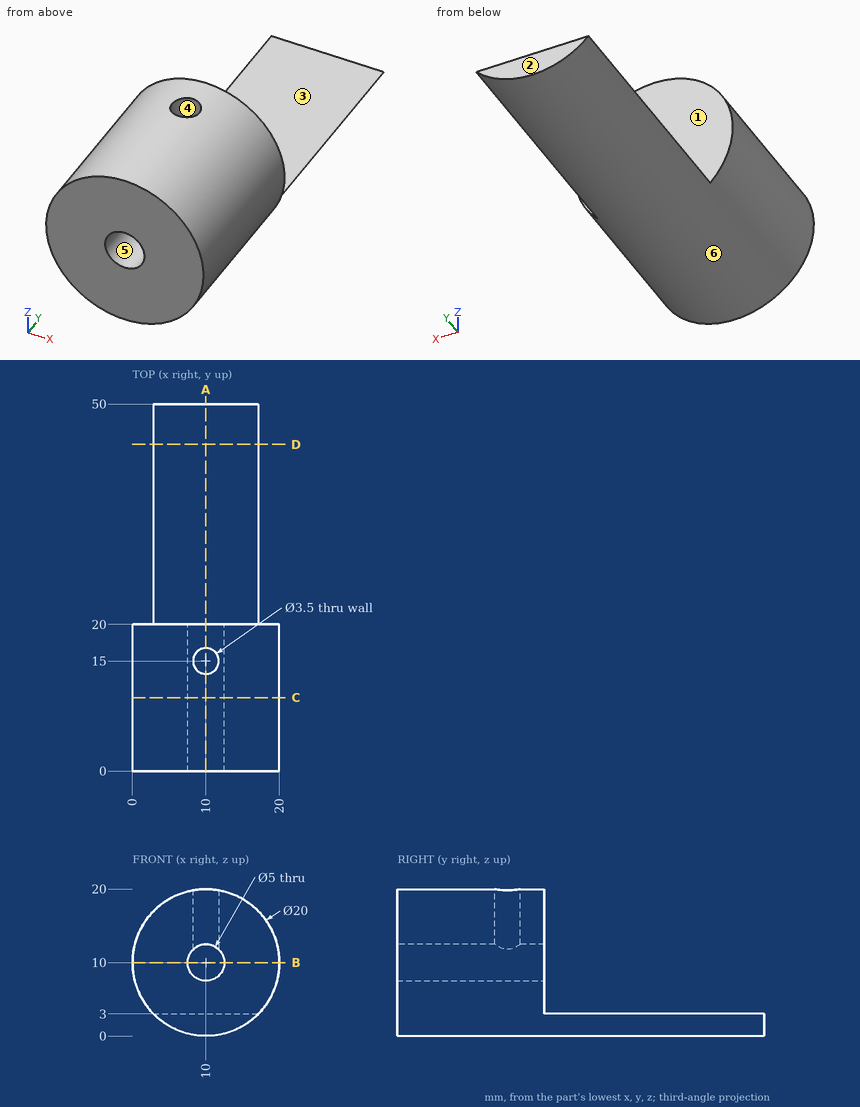
Print and shaded views of the part. All mm, measured from the part's lowest x, y and z. A direction names the side the tool comes from. Round coordinates to 2 decimals unless told otherwise and drop trailing zeros. Write each loop counter-clockwise with the first axis right and the second up, starting at its lowest first coordinate (ties: lowest second). Pieces come first, ordered by that corner, then holes. Notation, with made-up numbers: (39.25, -31.75) -> (72.25, -31.75) arc R20 ccw to (72.25, -25.75) -> close; hole circle Ø10 at (51, 63.5). An arc over 180 degrees is marked (long way). Answer in a Markdown table with one row per item. Add a question column.
Item 1: Saw through at B-B, the plane z = 10. Write the cut outline in (x, y).
Item 2: Drill centre lines: line 1 (X direction, y = 9, z = 10); line 2 (Y direction, x = 17, z = 11.5); line 3 (Z direction, x = 9.5, y = 4). Where is each one in solid material? Low to high. Write a range as from..to.
Item 3: Drop flat-ended pins along their axis: pin 1 Ø4 at (x, z) = (10, 10) entering from -Y; pin 2 Ø2 at (x, z) = (14.5, 13.5) entering from +Y; pin 3 Ø7 at (x, y) = (11, 40) entering from +Z; pin 4 Ø1 at (y, z) = (10, 14) entering from +X. Give the stop position or say it passes through.
Item 4: Mould opens along X. For the marked faces 3, 4, 5 and 6 say: pulls with the +X half, pulls with the -X half, needs draft (parallel to the pull), parting line crosses it, or undercut.
Item 5: Saw through at C-C, the plane y = 10. Write the cut outline in (x, z).
Item 6: Which spindle directions (+Z, -Z, +X, -X, +Y, -Y) get a long thin tool onto all of the face, cutting with end or side? Do the marked faces 1 and 2. Say none if no direction does.
Item 7: Saw through at A-A, the plane x = 10. Write the cut outline in (y, z), then the cut area to 3 significant figures.
Item 8: Saw through at D-D, the plane y = 44.5. Write the cut outline in (x, z), then the cut area to 3 significant figures.
Findings below:
| question | item | result |
|---|---|---|
| 1 | outline | (0, 0) -> (7.5, 0) -> (7.5, 20) -> (0, 20) -> close; (12.5, 0) -> (20, 0) -> (20, 20) -> (12.5, 20) -> close |
| 2 | line 1 | x = 0..7.5, 12.5..20 |
| 2 | line 2 | y = 0..20 |
| 2 | line 3 | z = 0.01..7.55, 12.45..19.99 |
| 3 | pin 1 | passes through |
| 3 | pin 2 | stops at y = 20 |
| 3 | pin 3 | stops at z = 3 |
| 3 | pin 4 | stops at x = 19.37 |
| 4 | face 3 | needs draft |
| 4 | face 4 | undercut |
| 4 | face 5 | undercut |
| 4 | face 6 | parting line crosses it |
| 5 | outline | circle Ø20 at (10, 10); hole circle Ø5 at (10, 10) |
| 6 | face 1 | +Z, +X, -X, +Y |
| 6 | face 2 | +Z, -Z, +X, -X, +Y |
| 7 | outline | (0, 0) -> (50, 0) -> (50, 3) -> (20, 3) -> (20, 7.5) -> (0, 7.5) -> close; (0, 12.5) -> (13.25, 12.5) -> (13.25, 20) -> (0, 20) -> close; (16.75, 12.5) -> (20, 12.5) -> (20, 20) -> (16.75, 20) -> close |
| 7 | area | 364 mm^2 |
| 8 | outline | (2.86, 3) arc R10 ccw to (17.14, 3) -> close |
| 8 | area | 29.5 mm^2 |
